Source: three-view drawing plus pictorial views. Frame: mm from the lowest corner of the part. Give positions to 0.01 mm unless a question says otherwise; leave off trailing zeros. Loops run counter-clockwise (first coordinate to the right, second up) from the corner with the lowest first, then second, coordinate; pieces in that order, holes last. Notation, with made-up numbers: (10.5, 11) - (21.5, 11) arc R17 cw to (21.5, 37) - close; hole circle Ø9 at (58, 76.25). An arc over 180 degrees is marked (long way). One line per item, written item: value.
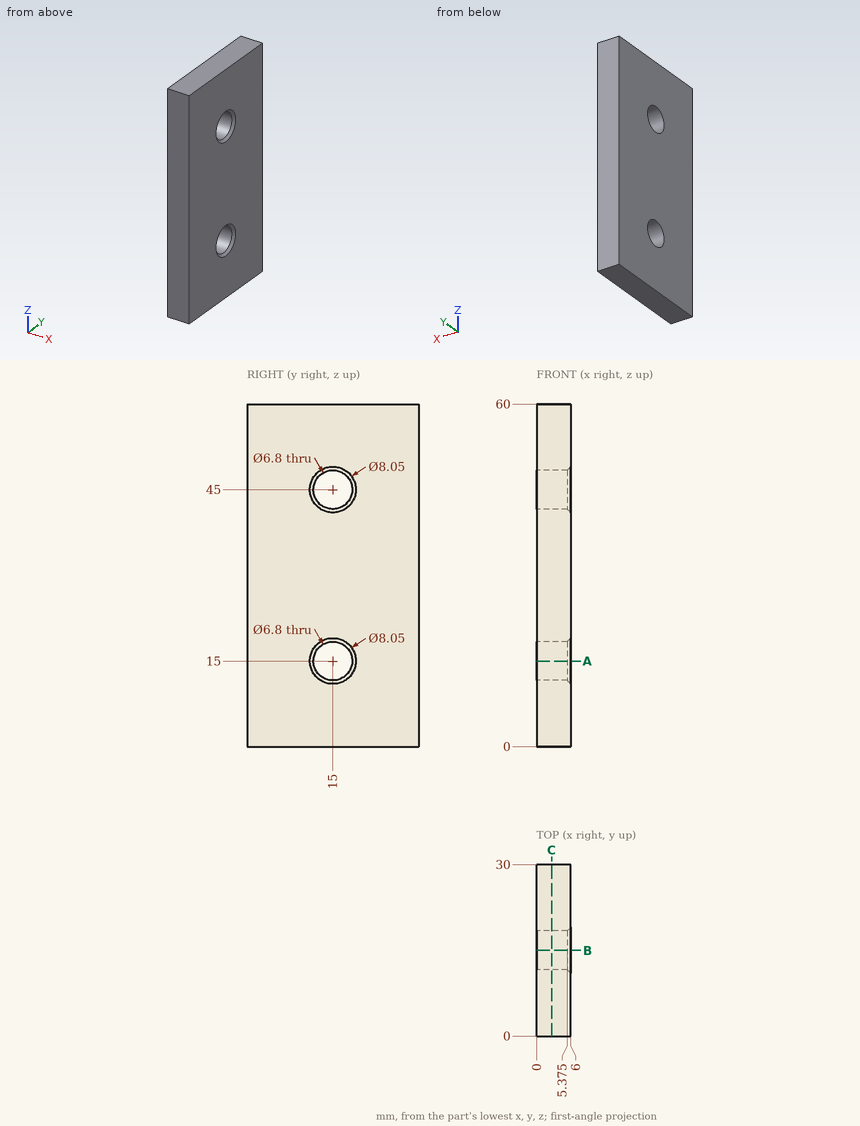
Item 1: Section C-C, the plane x = 2.65. Output: boundary loops of the cut face in (y, z).
Verdict:
outline: (0, 0) - (30, 0) - (30, 60) - (0, 60) - close; hole circle Ø6.8 at (15, 15); hole circle Ø6.8 at (15, 45)
Item 2: Pin query (flat end, axial travel): P1, Ø6, axis at y = 15, z = 15, coming from the -X side. Return the tip coordinate at first contact, or that it passes through.
Verdict:
P1: passes through
Item 3: Section A-A, the plane z = 15. Output: boundary loops of the cut face in (x, y) (3 decimals), and give its area (3 significant figures).
Verdict:
outline: (0, 0) - (6, 0) - (6, 10.975) - (5.375, 11.6) - (0, 11.6) - close; (0, 18.4) - (5.375, 18.4) - (6, 19.025) - (6, 30) - (0, 30) - close
area: 139 mm^2
Item 4: Material intervals for L1, parallel to Z at x = 1.25, y = 15; L2, parallel to Y at x = 2.6, z = 15; L3, parallel to Z at x = 2.2, y = 13, sorted ascending.
Verdict:
L1: z = 0 to 11.6, 18.4 to 41.6, 48.4 to 60
L2: y = 0 to 11.6, 18.4 to 30
L3: z = 0 to 12.25, 17.75 to 42.25, 47.75 to 60
Item 5: Section B-B, the plane y = 15. Output: boundary loops of the cut face in (x, z) (3 decimals).
Verdict:
outline: (0, 0) - (6, 0) - (6, 10.975) - (5.375, 11.6) - (0, 11.6) - close; (0, 18.4) - (5.375, 18.4) - (6, 19.025) - (6, 40.975) - (5.375, 41.6) - (0, 41.6) - close; (0, 48.4) - (5.375, 48.4) - (6, 49.025) - (6, 60) - (0, 60) - close
